Geometry: final body of the model. Coordinates: model frame, mm. Face numbers are marked on the shaded views. Give positions to 0.01 mm unless a question says otherwise; leave off trailing zeros. Write each loop counter-clockwise with the first axis right and the second up, starting at its lowest first coordinate (ties: lowest second). Pieces come first, ordered by that corner, then holes. Notation, with made-up numbers: M 47,-36 L 105,-36 A10 ccw 105,-25 Z; hole C -17.5,74.5 d1. An arc over 180 degrees is marked long. Use a Markdown table: item, result. Add a question column.
1) Section A-A on z = 6.5. Return the cut outline in (x, y), then the cut area to 3 significant figures.
2) Draft query along Z for the marked faces 1, 2 and 3. Return one class per face: +Z half, -Z half, draft (parallel to the pull), parting line (faces both ways), or undercut.
3) Pin query (flat end, axial travel): pin 1 (3 mm diameter, centred on x = 2.5, z = 17, fed in from +Y); pin 2 (1.8 mm diameter, centred on x = 1.5, z = 26, fed in from -Y); pin 3 (3 mm diameter, centred on x = 2.5, z = 26, fed in from +Y). Return the tip coordinate at first contact, or that it passes through.
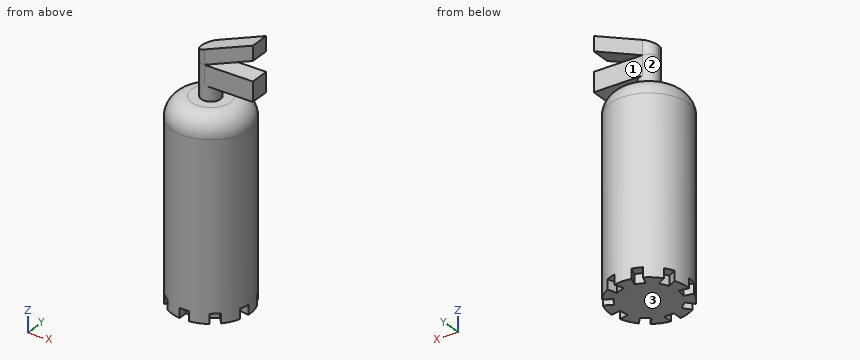
```python
from build123d import *

# Parameters (mm, degrees)
F0_R      = 4
F1_DEPTH  = 20
F2_R      = 2
F3_R      = 1
F4_DEPTH  = 1.5
F6_DEPTH  = 2
F8_DEPTH  = 2
F9_R      = 0.9999
F11_DEPTH = 1


# Not quite as in the source:
# - a fillet or chamfer is up to 0.001 mm smaller than in the source, because OpenCascade refuses the exact size


with BuildPart() as f1:
    # F0 (on Top) → F1 (new body)
    with BuildSketch(Plane.XY):
        Circle(F0_R)
    extrude(amount=F1_DEPTH)

    # F2
    f2_edges = [f1.edges().sort_by_distance(p)[0] for p in [
        (-4, 0, 20),
    ]]
    fillet(f2_edges, radius=F2_R)

    # F3 (on face) → F4 (join)
    with BuildSketch(Plane.XY.offset(20)):
        Circle(F3_R)
    extrude(amount=F4_DEPTH)

    # F5 (on face) → F6 (join)
    with BuildSketch(Plane.XY.offset(21.5)):
        with BuildLine():
            Line((5, 1), (0, 1))
            ThreePointArc((0, 1), (-1, 0), (0, -1))
            Line((0, -1), (5, -1))
            Line((5, -1), (5, 1))
        make_face()
    extrude(amount=F6_DEPTH)

    # F7 (on face) → F8 (join)
    with BuildSketch(Plane.XZ.offset(1)):
        Polygon((-1, 23.5), (0, 23.5), (5, 25.5), (5, 27), (-1, 24.6), align=None)
    extrude(amount=-F8_DEPTH)

    # F9 (radius 1 in the source; OpenCascade refuses exactly that, so slightly less here)
    f9_edges = [f1.edges().sort_by_distance(p)[0] for p in [
        (-1, -1, 24.05),
        (-1, 1, 24.05),
    ]]
    fillet(f9_edges, radius=F9_R)

    # F10 (on face) → F11 (cut)
    with BuildSketch(Plane(origin=(0, 0, 0), x_dir=(1, 0, 0), z_dir=(0, 0, -1))):
        Polygon((0.5, 4), (0, 4), (-0.5, 4), (-0.5, 3), (0.5, 3), align=None)
        Polygon((2.3113850506, 1.9767395245), (2.9541726603, 2.7427839676), (2.5711504387, 3.0641777725), (2.1881282172, 3.3855715773), (1.5453406075, 2.6195271342), align=None)
        Polygon((3.0412473479, 0.0285406565), (4.0260551009, 0.2021888342), (3.939231012, 0.6945927107), (3.8524069232, 1.1869965872), (2.8675991702, 1.0133484095), align=None)
        Polygon((2.3480762114, -1.9330127019), (3.2141016151, -2.4330127019), (3.4641016151, -2), (3.7141016151, -1.5669872981), (2.8480762114, -1.0669872981), align=None)
        Polygon((0.5562141196, -2.990087934), (0.8982342629, -3.9297805548), (1.3680805733, -3.7587704831), (1.8379268837, -3.5877604115), (1.4959067404, -2.6480677907), align=None)
        Polygon((-1.4959067404, -2.6480677907), (-1.8379268837, -3.5877604115), (-1.3680805733, -3.7587704831), (-0.8982342629, -3.9297805548), (-0.5562141196, -2.990087934), align=None)
        Polygon((-2.8480762114, -1.0669872981), (-3.7141016151, -1.5669872981), (-3.4641016151, -2), (-3.2141016151, -2.4330127019), (-2.3480762114, -1.9330127019), align=None)
        Polygon((-2.8675991702, 1.0133484095), (-3.8524069232, 1.1869965872), (-3.939231012, 0.6945927107), (-4.0260551009, 0.2021888342), (-3.0412473479, 0.0285406565), align=None)
        Polygon((-1.5453406075, 2.6195271342), (-2.1881282172, 3.3855715773), (-2.5711504387, 3.0641777725), (-2.9541726603, 2.7427839676), (-2.3113850506, 1.9767395245), align=None)
    extrude(amount=-F11_DEPTH, mode=Mode.SUBTRACT)


solid = f1.part
```
Found:
| question | item | result |
|---|---|---|
| 1 | outline | C 0,0 d8 |
| 1 | area | 50.3 mm² |
| 2 | face 1 | draft |
| 2 | face 2 | undercut |
| 2 | face 3 | -Z half |
| 3 | pin 1 | y = 3.87 |
| 3 | pin 2 | y = -1 |
| 3 | pin 3 | y = 1 |
